Can you work these out from the model? Positions are in its coordinate system, mm. Round coordinates to 2 decimals unless told otherwise and drop trailing zeros. Loops run counter-clockwise (first coordinate to the right, second up) from the corner with the lowest first, then second, coordinate; pieces in that order, holes last. Notation, with made-up numbers: (-15.75, 6) -> (7.25, 6) arc R5 cw to (7.25, 11) -> close; hole circle Ø1 at (3.25, -7.75). An arc over 180 degrees is marked (long way). Write each question's results on one line, items separated by ' | '.
from build123d import *

# Parameters (mm, degrees)
SKETCH1_W           = 95
SKETCH1_H           = 80
BOSS_EXTRUDE1_DEPTH = 3
SKETCH2_R           = 1.5
CUT_EXTRUDE1_DEPTH  = 3


with BuildPart() as part:
    # Sketch1 → Boss-Extrude1 (new body)
    with BuildSketch(Plane.XY):
        Rectangle(SKETCH1_W, SKETCH1_H)
    extrude(amount=BOSS_EXTRUDE1_DEPTH)

    # Sketch2 → Cut-Extrude1 (cut)
    with BuildSketch(Plane.XY.offset(3)):
        with Locations((-42.875692348, -32)):
            Circle(SKETCH2_R)
        with Locations((-18.825692348, -32)):
            Circle(SKETCH2_R)
        with Locations((-42.875692348, 32)):
            Circle(SKETCH2_R)
        with Locations((-18.825692348, 32)):
            Circle(SKETCH2_R)
        with Locations((-42.5, 10.92769595)):
            Circle(SKETCH2_R)
        with Locations((-25.5, 10.92769595)):
            Circle(SKETCH2_R)
        with Locations((-42.5, -15.07230405)):
            Circle(SKETCH2_R)
        with Locations((-25.5, -15.07230405)):
            Circle(SKETCH2_R)
        with Locations((42.5, -12.5)):
            Circle(SKETCH2_R)
        with Locations((42.5, 12.5)):
            Circle(SKETCH2_R)
        with Locations((18.909687324, 32)):
            Circle(SKETCH2_R)
        with Locations((42.959687324, 32)):
            Circle(SKETCH2_R)
        with Locations((18.909687324, -32)):
            Circle(SKETCH2_R)
        with Locations((42.959687324, -32)):
            Circle(SKETCH2_R)
    extrude(amount=-CUT_EXTRUDE1_DEPTH, mode=Mode.SUBTRACT)


solid = part.part
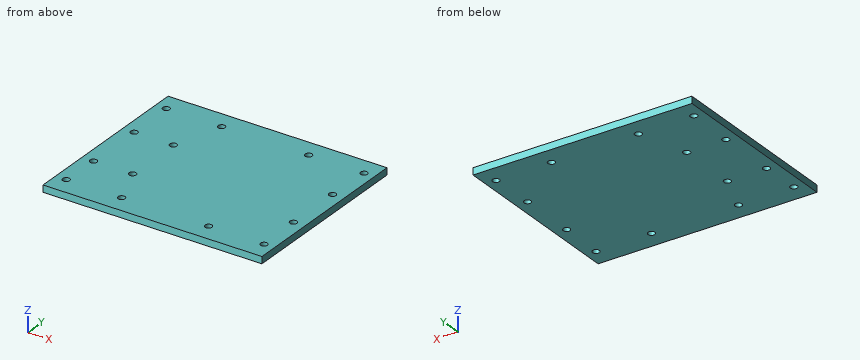
1. Will this pin go through, and if not, where does the flat tip stop? pin 1 (12 mm diameter, centred on x = 1, y = 6.5, fed in from -Z).
Final values:
pin 1: z = 0
2. If we section it at A-A (y = -32): List the corners of the cut face in (x, z) for me.
Final values:
outline: (-47.5, 0) -> (-44.38, 0) -> (-44.38, 3) -> (-47.5, 3) -> close; (-41.38, 0) -> (-20.33, 0) -> (-20.33, 3) -> (-41.38, 3) -> close; (-17.33, 0) -> (17.41, 0) -> (17.41, 3) -> (-17.33, 3) -> close; (20.41, 0) -> (41.46, 0) -> (41.46, 3) -> (20.41, 3) -> close; (44.46, 0) -> (47.5, 0) -> (47.5, 3) -> (44.46, 3) -> close
3. Please list where these lines run through material, in increasing order: line 1 (Y direction, x = -19, z = 0.7); line 2 (Y direction, x = -25.5, z = 1.05); line 3 (Y direction, x = -42, z = 2.8). Write a range as from..to.
Final values:
line 1: -40..-33.49, -30.51..30.51, 33.49..40 | line 2: -40..-16.57, -13.57..9.43, 12.43..40 | line 3: -40..-33.22, -30.78..-16.49, -13.66..9.51, 12.34..30.78, 33.22..40
4. If we section it at D-D (x = -42.5): List the corners of the cut face in (y, z) for me, then the cut area to 3 significant figures.
Final values:
outline: (-40, 0) -> (-33.45, 0) -> (-33.45, 3) -> (-40, 3) -> close; (-30.55, 0) -> (-16.57, 0) -> (-16.57, 3) -> (-30.55, 3) -> close; (-13.57, 0) -> (9.43, 0) -> (9.43, 3) -> (-13.57, 3) -> close; (12.43, 0) -> (30.55, 0) -> (30.55, 3) -> (12.43, 3) -> close; (33.45, 0) -> (40, 0) -> (40, 3) -> (33.45, 3) -> close | area: 205 mm2
5. If we section it at B-B (x = -25.5): List the corners of the cut face in (y, z) for me, then the cut area to 3 significant figures.
Final values:
outline: (-40, 0) -> (-16.57, 0) -> (-16.57, 3) -> (-40, 3) -> close; (-13.57, 0) -> (9.43, 0) -> (9.43, 3) -> (-13.57, 3) -> close; (12.43, 0) -> (40, 0) -> (40, 3) -> (12.43, 3) -> close | area: 222 mm2
6. If we section it at C-C (y = -12.5): List the corners of the cut face in (x, z) for me.
Final values:
outline: (-47.5, 0) -> (41, 0) -> (41, 3) -> (-47.5, 3) -> close; (44, 0) -> (47.5, 0) -> (47.5, 3) -> (44, 3) -> close
